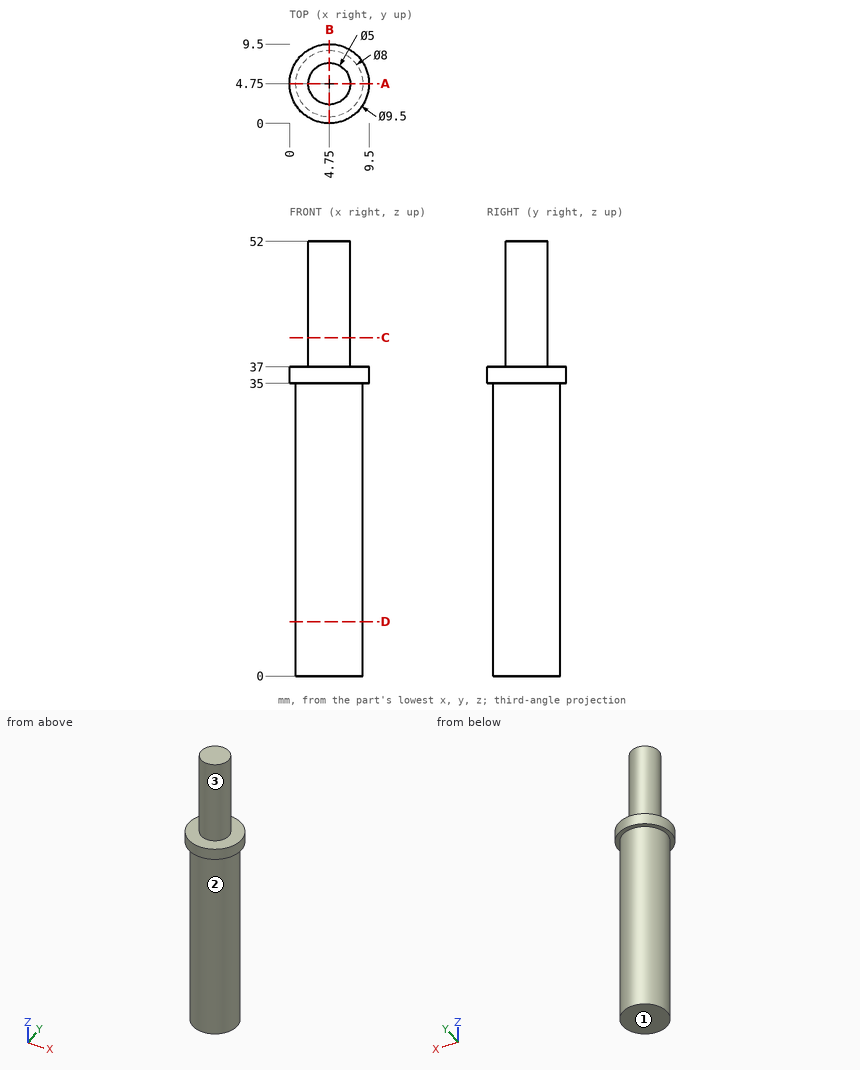
Part print with two shaded views. Sizes in mm from the minimum x, y, z corner. A direction names the side the tool comes from. Round coordinates to 2 decimals unless told otherwise and drop trailing zeros. Loops run counter-clockwise (first coordinate to the right, second up) from the corner with the lowest first, then second, coordinate; pieces in that order, holes last. Notation, with made-up numbers: M 58,12.25 L 103,12.25 A34 ccw 103,43.25 Z; hole C -26.75,74 d9. An arc over 180 degrees is marked long. Put each result on its own line as item: value. Start each with the question number.
Item 1: Cut at D-D (z = 6.5). List the corners of the cut face in (x, y), then the cut area to 3 significant figures.
Item 2: 3-axis set-ups, long thin cutter, end or side, ignore diameter. For the marked faces 1, 2 and 3: which of +Z, -Z, +X, -X, +Y, -Y reach the whole face in a straight line?
Item 3: Cut at A-A (y = 4.75). List the corners of the cut face in (x, z).
Item 4: Drill centre lines: line 1 along X through (y, z) = (4.5, 9.5); line 2 along Z through (x, y) = (2.5, 7.5). Where is each one in solid material? Low to high.
Item 5: Drop flat-ended pins along their axis: P1, Ø2, axis at x = 5, z = 26.5, coming from the -Y side; P2, Ø1.5, axis at y = 1, z = 13.5, coming from the +X side. Give the stop position or say it passes through.
Item 6: Cut at C-C (z = 40.5). List the corners of the cut face in (x, y).
Answer block:
1. outline: C 4.75,4.75 d8
1. area: 50.3 mm2
2. face 1: -Z, +X, -X, +Y, -Y
2. face 2: -Z
2. face 3: +Z
3. outline: M 0,35 L 0.75,35 L 0.75,0 L 8.75,0 L 8.75,35 L 9.5,35 L 9.5,37 L 7.25,37 L 7.25,52 L 2.25,52 L 2.25,37 L 0,37 Z
4. line 1: 0.76 to 8.74
4. line 2: 0 to 37
5. P1: y = 0.75
5. P2: x = 7.4
6. outline: C 4.75,4.75 d5
